Autodesk Inventor part; units mm, degrees
ref_plane "YZ Plane" through (0, 0, 0) normal (1, 0, 0) x (0, 1, 0)
ref_plane "XZ Plane" through (0, 0, 0) normal (0, 1, 0) x (-1, 0, 0)
ref_plane "XY Plane" through (0, 0, 0) normal (0, 0, 1) x (1, 0, 0)
sketch "Sketch1" plane through (0, 0, 0) normal (0, 0, 1) x (1, 0, 0)
  point P0 (0, 0)
sketch "Sketch2" plane through (0, 0, 0) normal (0, 1, 0) x (-1, 0, 0)
  line L0 (3.175, 0) -> (44.45, 0)
  circle A0 centre (44.45, 19.05) radius 9.525
  arc A1 (44.45, 0) -> (25.4113, 18.3929) centre (44.45, 19.05) ccw
  line L1 (0, 3.175) -> (0, 12.065)
  circle A2 centre (10.16, 7.62) radius 3.175
  line L2 (3.175, 15.24) -> (22.6099, 15.24)
  arc A3 (3.175, 15.24) -> (0, 12.065) centre (3.175, 12.065) ccw
  arc A4 (0, 3.175) -> (3.175, 0) centre (3.175, 3.175) ccw
  arc A5 (22.6099, 15.24) -> (25.4113, 18.3929) centre (22.2363, 18.3929) ccw
  point P0 (0, 0)
  point P1 (0, 15.24)
  dimension "d1" = 44.45
  dimension "d3" = 19.05
  dimension "d4" = 38.1
  dimension "d5" = 15.24
  dimension "d7" = 6.35
  dimension "d8" = 3.175
  dimension "d11" = 3.175
extrude "Extrusion1" add sketch "Sketch2" against normal blind 25.4
ref_plane "Work Plane5" through (-44.45, 0, 38.1) normal (0, 0, 1) x (1, 0, 0)
sketch "Sketch5" plane through (-44.45, 0, 38.1) normal (0, 0, 1) x (1, 0, 0)
  line L0 (-19.05, 0) -> (-19.05, -25.4)
  circle A0 centre (0, -12.7) radius 3.175
  point P0 (44.45, 0)
  point P1 (0, -25.4)
  point P2 (19.0387, -25.4)
  dimension "d21" = 6.35
extrude "Extrusion2" cut sketch "Sketch5" against normal through all
properties part number "Assignment 2.6 - Shaft Guide"
The listing builds one solid part. Answer for the finished solid, in the listing's coordinates (mm). A direction names the side the tool comes from. Give positions to 0.01 mm unless a question says otherwise; leave off trailing zeros. Loops run counter-clockwise (first coordinate to the right, second up) from the corner with the lowest first, then second, coordinate; pieces in that order, holes last. Notation, with made-up numbers: (67.25, 32) - (75.25, 32) arc R20 cw to (75.25, 50) - close; hole circle Ø6 at (-4.75, -23.75). An arc over 180 degrees is marked (long way). Return JSON: item names as keys, results as strings. Group by question number.
1. Which of the six approach directions +Z, -Z, +X, -X, +Y, -Y give full straight-line access (tool end or side, diameter ignored) to faces 4 (the flat face through (-13, -13, 15.24)), 5 (the cylindrical face through (-48.85, -12.52, 10.6))?
2. Find section C-C (y = -17.5). Write down the section's boundary in (x, z) (3 decimals), then the cut area to 3 significant figures.
3. Find section A-A (z = 19.05). Write down the section's boundary in (x, y) (3 decimals), then the cut area to 3 significant figures.
4. Find section D-D (z = 7.62). Write down the section's boundary in (x, y) (3 decimals).
5. Determine the mould class of faces 1 (the cylindrical face through (-41.52, -13.92, 33.14)), 2 (the cylindrical face through (-0.95, -12.52, 14.33)), 3 (the flat face through (-31, 0, 15)) for opening direction X: pulls with the +X half, pulls with the -X half, needs draft (parallel to the pull), parting line crosses it, or undercut.
6. Straight lines are drawn through the part: line 1 (Y direction, x = -44.45, z = 2.5) (3 decimals); line 2 (Z direction, x = -10.16, y = -14) (3 decimals); line 3 (X direction, y = -9.5, z = 19). For each, find the intervals that lie inside material, in ascending order. Write a range as [from, to].
7. Given pin 1 Ø6 at (y, z) = (-9.5, 28) entering from +X; pin 2 Ø10 at (x, y) = (-19.5, -15.5) entering from +Z; pin 3 Ø2 at (y, z) = (-7.5, 32.5) entering from +X, each flat-ended and moving along its own axis, determine where each tip first touches the part or whether it passes through.
8. Find section B-B (y = -12.7). Write down the section's boundary in (x, z) (3 decimals).
Verdict:
{
 "1": {"face 4": "+Z, +X, +Y, -Y", "face 5": "+Y, -Y"},
 "2": {"outline": "(-44.45, 0) - (-3.175, 0) arc R3.175 ccw to (0, 3.175) - (0, 12.065) arc R3.175 ccw to (-3.175, 15.24) - (-22.61, 15.24) arc R3.175 cw to (-25.411, 18.393) arc R19.05 ccw (long way) to start; hole circle Ø19.05 at (-44.45, 19.05); hole circle Ø6.35 at (-10.16, 7.62)", "area": "1,290 mm^2"},
 "3": {"outline": "(-63.5, -25.4) - (-53.975, -25.4) - (-53.975, 0) - (-63.5, 0) - close; (-34.925, -25.4) - (-25.4, -25.4) - (-25.4, 0) - (-34.925, 0) - close", "area": "484 mm^2"},
 "4": {"outline": "(-59.69, -25.4) - (-13.335, -25.4) - (-13.335, 0) - (-59.69, 0) - close; (-6.985, -25.4) - (0, -25.4) - (0, 0) - (-6.985, 0) - close; hole circle Ø6.35 at (-44.45, -12.7)"},
 "5": {"face 1": "undercut", "face 2": "pulls with the +X half", "face 3": "needs draft"},
 "6": {"line 1": "y = [-25.4, -15.875], [-9.525, 0]", "line 2": "z = [0, 4.445], [10.795, 15.24]", "line 3": "x = [-63.5, -53.97], [-34.93, -25.4]"},
 "7": {"pin 1": "stops at x = -26.35", "pin 2": "stops at z = 16.17", "pin 3": "stops at x = -30.03"},
 "8": {"outline": "(-47.625, 0.266) - (-47.625, 10.07) arc R9.525 cw to (-47.625, 28.03) - (-47.625, 37.834) arc R19.05 ccw to start; (-41.275, 0) - (-3.175, 0) arc R3.175 ccw to (0, 3.175) - (0, 12.065) arc R3.175 ccw to (-3.175, 15.24) - (-22.61, 15.24) arc R3.175 cw to (-25.411, 18.393) arc R19.05 ccw to (-41.275, 37.834) - (-41.275, 28.03) arc R9.525 cw to (-41.275, 10.07) - close; hole circle Ø6.35 at (-10.16, 7.62)"}
}
